Input: part model. Units: mm. Frame: model coordinates. A direction names the side the tool comes from. Coordinates: 2 decimals unless noted, no trailing zeros. Write each loop counter-clockwise with the first axis right and the second up, starting at its lowest first coordinate (ties: lowest second). Pieces come first, ordered by that corner, then holes. Notation, with made-up numbers: (37, 9.25) - (78, 9.25) arc R6 ccw to (78, 16.25) - close; hole circle Ø11 at (-39, 61). An arc over 180 degrees is marked (long way). One line per question, with ' | ' between items. Start each with the question number.
1) Section query A-A on z = -33.9. Return loops of the section in (x, y), and give its area (3 significant figures).
2) Line query: line 1 (X direction, y = 0.2, z = -33.9); line 2 (Z direction, x = 16, y = 1.35); line 3 (Z direction, x = -16, y = 0.4). Output: solid intervals per line, ascending.
3) First-contact query: P1, Ø2, axis at x = -16.5, z = -34, coming from the +Y side. Flat tip, straight axial feed; report the tip coordinate or a pass-through.
4) Section query B-B on y = 1.2. Return loops of the section in (x, z).
5) Section query C-C on x = 16. Return loops of the section in (y, z).
6) Draft query along Z for faces 3 (the flat face through (0, 1, -36.9)), 4 (the flat face through (-19, 1, 1)), 5 (the cylindrical face through (-16, 1, 36)), 6 (the flat face through (0, 1, 36.9)). Return one class per face: released by +Z, released by -Z, zero draft, split by the parting line, or undercut.
7) Reachability of faces 1 (the flat face through (17, 0.8, -33)), 2 (the cylindrical face through (16.954, 0.406, -34.2)) from +Z, -Z, +X, -X, +Y, -Y: full face, straight path, thin tool, end or side. Return the list, or none.
```python
from build123d import *

# Parameters (mm, degrees)
SKETCH1_W           = 38
SKETCH1_H           = 73.8
BOSS_EXTRUDE1_DEPTH = 1.8
SKETCH2_R           = 1
CUT_EXTRUDE1_DEPTH  = 2.8
SKETCH3_R           = 2.1
CUT_EXTRUDE2_DEPTH  = 1
FILLET1_R           = 1


with BuildPart() as part:
    # Sketch1 → Boss-Extrude1 (new body)
    with BuildSketch(Plane(origin=(0, 0, 0), x_dir=(1, 0, 0), z_dir=(0, 1, 0))):
        Rectangle(SKETCH1_W, SKETCH1_H)
    extrude(amount=BOSS_EXTRUDE1_DEPTH)

    # Sketch2 → Cut-Extrude1 (cut, through all)
    with BuildSketch(Plane(origin=(0, 1.8, 0), x_dir=(1, 0, 0), z_dir=(0, 1, 0))):
        with Locations((-16, 33.9)):
            Circle(SKETCH2_R)
        with Locations((16, 33.9)):
            Circle(SKETCH2_R)
    cut_extrude1 = extrude(amount=-CUT_EXTRUDE1_DEPTH, mode=Mode.SUBTRACT)

    # Sketch3 → Cut-Extrude2 (cut)
    with BuildSketch(Plane(origin=(0, 1.8, 0), x_dir=(1, 0, 0), z_dir=(0, 1, 0))):
        with Locations((-16, 33.9)):
            Circle(SKETCH3_R)
        with Locations((16, 33.9)):
            Circle(SKETCH3_R)
    cut_extrude2 = extrude(amount=-CUT_EXTRUDE2_DEPTH, mode=Mode.SUBTRACT)

    # Mirror1: Cut-Extrude1, Cut-Extrude2 across plane
    add(cut_extrude1.mirror(Plane.XY), mode=Mode.SUBTRACT)
    add(cut_extrude2.mirror(Plane.XY), mode=Mode.SUBTRACT)

    # Fillet1
    fillet1_edges = [part.edges().sort_by_distance(p)[0] for p in [
        (19, 0.9, 36.9),
        (-19, 0.9, 36.9),
        (-19, 0.9, -36.9),
        (19, 0.9, -36.9),
    ]]
    fillet(fillet1_edges, radius=FILLET1_R)


solid = part.part
```
Answer key:
1) outline: (-19, 0) - (-17, 0) - (-17, 0.8) - (-18.1, 0.8) - (-18.1, 1.8) - (-19, 1.8) - close; (-15, 0) - (15, 0) - (15, 0.8) - (13.9, 0.8) - (13.9, 1.8) - (-13.9, 1.8) - (-13.9, 0.8) - (-15, 0.8) - close; (17, 0) - (19, 0) - (19, 1.8) - (18.1, 1.8) - (18.1, 0.8) - (17, 0.8) - close | area: 56.8 mm²
2) line 1: -19 to -17, -15 to 15, 17 to 19 | line 2: -36.9 to -36, -31.8 to 31.8, 36 to 36.9 | line 3: -36.9 to -34.9, -32.9 to 32.9, 34.9 to 36.9
3) P1: y = 0.8
4) outline: (-19, -35.9) arc R1 ccw to (-18, -36.9) - (18, -36.9) arc R1 ccw to (19, -35.9) - (19, 35.9) arc R1 ccw to (18, 36.9) - (-18, 36.9) arc R1 ccw to (-19, 35.9) - close; hole circle Ø4.2 at (-16, -33.9); hole circle Ø4.2 at (-16, 33.9); hole circle Ø4.2 at (16, -33.9); hole circle Ø4.2 at (16, 33.9)
5) outline: (0, -36.9) - (1.8, -36.9) - (1.8, -36) - (0.8, -36) - (0.8, -34.9) - (0, -34.9) - close; (0, -32.9) - (0.8, -32.9) - (0.8, -31.8) - (1.8, -31.8) - (1.8, 31.8) - (0.8, 31.8) - (0.8, 32.9) - (0, 32.9) - close; (0, 34.9) - (0.8, 34.9) - (0.8, 36) - (1.8, 36) - (1.8, 36.9) - (0, 36.9) - close
6) face 3: released by -Z | face 4: zero draft | face 5: undercut | face 6: released by +Z
7) face 1: +Y | face 2: +Y, -Y
